Geometry check sheet. Reference: the model listing, model coordinates, mm. A direction names the side the tool comes from. Coordinates: 2 decimals unless noted, no trailing zeros. Write each loop counter-clockwise with the first axis right and the second up, starting at its lowest first coordinate (ties: lowest second). Pieces come first, ordered by that corner, then holes. Notation, with made-up numbers: (69, -15.75) - (107, -15.75) arc R15 ccw to (107, 11.25) - close; hole circle Ø6 at (51.25, -9). An arc over 180 degrees is marked (long way). Answer as a JSON object with one key per item and string values. Group by question number.
from build123d import *

# Parameters (mm, degrees)
BOSS_EXTRUDE1_DEPTH = 27.686
SKETCH2_W           = 29.921903197
SKETCH2_H           = 4.572
CUT_EXTRUDE1_DEPTH  = 13.843
SKETCH3_OUTSIDE_W   = 46.952
SKETCH3_OUTSIDE_H   = 142.689
CUT_EXTRUDE2_DEPTH  = 27.686


with BuildPart() as part:
    # Sketch1 → Boss-Extrude1 (new body)
    with BuildSketch(Plane(origin=(0, 0, 0), x_dir=(1, 0, 0), z_dir=(0, 1, 0))):
        with BuildLine():
            Line((-10.156518422, -0.265957795), (-7.828589994, -89.165957795))
            ThreePointArc((-7.828589994, -89.165957795), (0, -106.245464925), (7.828589994, -89.165957795))
            Line((7.828589994, -89.165957795), (10.156518422, -0.265957795))
            ThreePointArc((10.156518422, -0.265957795), (0, 10.16), (-10.156518422, -0.265957795))
        make_face()
    extrude(amount=BOSS_EXTRUDE1_DEPTH)

    # Sketch2 → Cut-Extrude1 (cut, symmetric)
    with BuildSketch(Plane(origin=(0, 0, 0.265957795), x_dir=(-1, 0, 0), z_dir=(0, 0, -1))):
        with Locations((1.107435291, 13.843)):
            Rectangle(SKETCH2_W, SKETCH2_H)
    extrude(amount=CUT_EXTRUDE1_DEPTH, both=True, mode=Mode.SUBTRACT)

    # Sketch3 outside → Cut-Extrude2 (cut)
    with BuildSketch(Plane.XZ):
        with Locations((0, 48.0425)):
            Rectangle(SKETCH3_OUTSIDE_W, SKETCH3_OUTSIDE_H)
        with BuildLine():
            Line((10.156518422, 0.265957795), (7.828589994, 89.165957795))
            ThreePointArc((7.828589994, 89.165957795), (0, 106.245464925), (-7.828589994, 89.165957795))
            Line((-7.828589994, 89.165957795), (-10.156518422, 0.265957795))
            ThreePointArc((-10.156518422, 0.265957795), (0, -10.16), (10.156518422, 0.265957795))
        make_face(mode=Mode.SUBTRACT)
        with BuildLine():
            Line((-1.397467487, 92.180775304), (-3.808694408, 0.099734173))
            ThreePointArc((-3.808694408, 0.099734173), (0, -3.81), (3.808694408, 0.099734173))
            Line((3.808694408, 0.099734173), (1.397467487, 92.180775304))
            ThreePointArc((1.397467487, 92.180775304), (0, 91.927632861), (-1.397467487, 92.180775304))
        make_face()
    extrude(amount=-CUT_EXTRUDE2_DEPTH, mode=Mode.SUBTRACT)


solid = part.part
(1) Section check A-A (x = 0). Record the cut outline in (y, z), and give its area (3 significant figures).
(2) Gauge pin test, flat ends, axial feed: pin 1 (3 mm diameter, centred on y = 22, z = 70, fed in from -X); pin 2 (1.5 mm diameter, centred on y = 8, z = 42, fed in from -X); pin 3 (5 mm diameter, centred on x = 5.5, y = 14, fed in from -Z); pin 4 (3 mm diameter, centred on x = 0.5, z = 22, fed in from -Y) (3 decimals). Record the tip position at first contact, or that the pin passes through.
(3) Section check B-B (y = 3.75). Record the cut outline in (x, z).
(4) Section check C-C (z = -2). Record the cut outline in (x, y).
(5) Draft check along Y on faces 4 (the face through (-7, 14, 14.109)), 5 (the face through (0.227, 5.698, -10.157)), 6 (the face through (4, 27.686, 47)). Enter one of: +Y half, -Y half, draft (parallel to the pull), parting line (faces both ways), or undercut.
(6) Section check D-D (z = 64.5). Record the cut outline in (x, y).
(7) Material ranges on L1, parallel to Y at x = 4, z = 7.5; L2, parallel to X at y = 23, z = 31; L3, parallel to X at y = 10.25, z = 63, recorded low to high. Write a range as [from, to].
(8) Set-up check for faces 1 (the face through (4, 0, 47)), 2 (the face through (5, 11.557, 2)), 3 (the face through (-0.09, 5.7, -3.81)): record each of +Z, -Z, +X, -X, +Y, -Y from which the full face is reachable in a straight line by a thin tool's end or side.
Conclusion:
{
 "1": {"outline": "(0, -10.16) - (11.56, -10.16) - (11.56, -3.81) - (0, -3.81) - close; (0, 91.93) - (27.69, 91.93) - (27.69, 106.25) - (0, 106.25) - close; (16.13, -10.16) - (27.69, -10.16) - (27.69, -3.81) - (16.13, -3.81) - close", "area": "543 mm^2"},
 "2": {"pin 1": "stops at x = -8.37", "pin 2": "stops at x = -9.08", "pin 3": "stops at z = -9.26", "pin 4": "passes through"},
 "3": {"outline": "(-10.16, 0.27) arc R10.16 ccw (long way) to (10.16, 0.27) - (7.83, 89.17) arc R10.33 ccw (long way) to (-7.83, 89.17) - close; hole (-3.81, 0.1) arc R3.81 ccw (long way) to (3.81, 0.1) - (1.4, 92.18) arc R3.98 cw to (-1.4, 92.18) - close"},
 "4": {"outline": "(-9.96, 0) - (-3.24, 0) - (-3.24, 11.56) - (-9.96, 11.56) - close; (-9.96, 16.13) - (-3.24, 16.13) - (-3.24, 27.69) - (-9.96, 27.69) - close; (3.24, 0) - (9.96, 0) - (9.96, 11.56) - (3.24, 11.56) - close; (3.24, 16.13) - (9.96, 16.13) - (9.96, 27.69) - (3.24, 27.69) - close"},
 "5": {"face 4": "undercut", "face 5": "draft", "face 6": "+Y half"},
 "6": {"outline": "(-8.47, 0) - (-2.12, 0) - (-2.12, 27.69) - (-8.47, 27.69) - close; (2.12, 0) - (8.47, 0) - (8.47, 27.69) - (2.12, 27.69) - close"},
 "7": {"L1": "y = [0, 11.56], [16.13, 27.69]", "L2": "x = [-9.35, -3], [3, 9.35]", "L3": "x = [-8.51, -2.16], [2.16, 8.51]"},
 "8": {"face 1": "+Z, -Z, +X, -X, -Y", "face 2": "-Z, +X, -X", "face 3": "+Y, -Y"}
}
